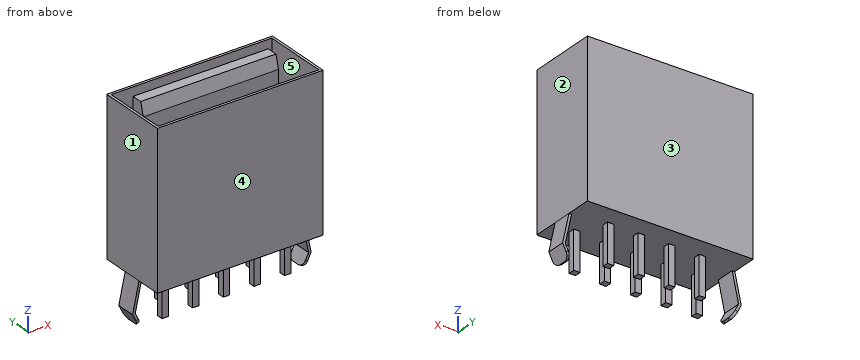
```python
from build123d import *

# Parameters (mm, degrees)
SKETCH_1_W          = 13
SKETCH_1_H          = 5.5
EXTRUDE_1_DEPTH     = 12
SKETCH_2_W          = 12.6
SKETCH_2_H          = 5.1
CUT_EXTRUDE_1_DEPTH = 10
SKETCH_5_W          = 10.6
SKETCH_5_H          = 1.1
EXTRUDE_3_DEPTH     = 10
CHAMFER_1_SIZE      = 1
CHAMFER_1_SIZE2     = 0.267949192
SKETCH_13_W         = 0.5
SKETCH_13_H         = 0.5
EXTRUDE_7_DEPTH     = 3
THICKEN_START       = -0.75
THICKEN_1_DEPTH     = 1.5
THICKEN_2_DEPTH     = 1.5
FILLET_2_R          = 0.5


# Read off the part's stored shape, not the designer's step: 加厚1, 加厚2
with BuildPart() as part:
    # 草图1 → 凸台-拉伸1 (new body)
    with BuildSketch(Plane.XY):
        Rectangle(SKETCH_1_W, SKETCH_1_H)
    extrude(amount=EXTRUDE_1_DEPTH)

    # 草图2 → 切除-拉伸1 (cut)
    with BuildSketch(Plane.XY.offset(12)):
        Rectangle(SKETCH_2_W, SKETCH_2_H)
    extrude(amount=-CUT_EXTRUDE_1_DEPTH, mode=Mode.SUBTRACT)

    # 草图5 → 凸台-拉伸3 (add)
    with BuildSketch(Plane.XY.offset(2)):
        with Locations((0, 1)):
            Rectangle(SKETCH_5_W, SKETCH_5_H)
    extrude(amount=EXTRUDE_3_DEPTH)

    # 倒角1
    chamfer_1_edges = [part.edges().sort_by_distance(p)[0] for p in [
        (0, 0.45, 12),
    ]]
    chamfer_1_side = [part.faces().sort_by_distance(p)[0] for p in [
        (0, 0.45, 7),
    ]]
    chamfer(chamfer_1_edges, length=CHAMFER_1_SIZE, length2=CHAMFER_1_SIZE2, reference=chamfer_1_side[0])

    # 草图13 → 凸台-拉伸7 (add)
    with BuildSketch(Plane(origin=(0, 0, 0), x_dir=(-1, 0, 0), z_dir=(0, 0, -1))):
        with Locations((-3.6, 1)):
            Rectangle(SKETCH_13_W, SKETCH_13_H)
        with Locations((-1.2, 1)):
            Rectangle(SKETCH_13_W, SKETCH_13_H)
        with Locations((1.2, 1)):
            Rectangle(SKETCH_13_W, SKETCH_13_H)
        with Locations((3.6, 1)):
            Rectangle(SKETCH_13_W, SKETCH_13_H)
        with Locations((-2.4, -0.993127881)):
            Rectangle(SKETCH_13_W, SKETCH_13_H)
        with Locations((-4.8, -0.993127881)):
            Rectangle(SKETCH_13_W, SKETCH_13_H)
        with Locations((0, -0.993127881)):
            Rectangle(SKETCH_13_W, SKETCH_13_H)
        with Locations((2.4, -0.993127881)):
            Rectangle(SKETCH_13_W, SKETCH_13_H)
        with Locations((4.8, -0.993127881)):
            Rectangle(SKETCH_13_W, SKETCH_13_H)
    extrude(amount=EXTRUDE_7_DEPTH)

    # 加厚1 outline → 加厚1 (add)
    with BuildSketch(Plane(origin=(0, 0, 0), x_dir=(1, 0, 0), z_dir=(0, 1, 0)).offset(THICKEN_START)):
        Polygon((6.78959064, 2.273605125), (6.295328656, 0), (6.5, 0), (7, 2.3), (6.5, 3.3), (6.321114562, 3.210557281), align=None)
    extrude(amount=THICKEN_1_DEPTH)

    # 加厚2 outline → 加厚2 (add)
    with BuildSketch(Plane(origin=(0, 0, 0), x_dir=(1, 0, 0), z_dir=(0, 1, 0)).offset(THICKEN_START)):
        Polygon((-6.5, 0), (-6.295328656, 0), (-6.78959064, 2.273605125), (-6.321114562, 3.210557281), (-6.5, 3.3), (-7, 2.3), align=None)
    extrude(amount=THICKEN_2_DEPTH)

    # 圆角2
    fillet_2_edges = [part.edges().sort_by_distance(p)[0] for p in [
        (6.410557281, -0.75, -3.25527864),
        (6.410557281, 0.75, -3.25527864),
        (-6.410557281, -0.75, -3.25527864),
        (-6.410557281, 0.75, -3.25527864),
    ]]
    fillet(fillet_2_edges, radius=FILLET_2_R)


solid = part.part
```
Source: CAD feature listing. Evaluate the final solid. Frame: model axes, mm. Face numbers are marked on the shaded views. A direction names the side the tool comes from. Round coordinates to 2 decimals unless told otherwise and drop trailing zeros. Loops run counter-clockwise (first coordinate to the right, second up) from the corner with the lowest first, then second, coordinate; pieces in that order, holes last.
1. Mould query, pull axis Y, two halves, no side actions, for the marked faces 3, 4 and 5. Classes: released by +Y, released by -Y, zero draft, split by the parting line, or undercut.
2. Access query for the marked faces 1 and 2. Directions: +Z, -Z, +X, -X, +Y, -Y. A direction counts if a zero-diameter tool reaches every point of the face in a straight line with its end or side. Return the directions, or none.
3. Section query C-C on y = -2.35. Output: boundary loops of the cut face in (x, z), and give its area (3 significant figures).
4. Section query B-B on x = 0.5. Output: boundary loops of the cut face in (y, z).
5. Section query A-A on z = 8. Output: boundary loops of the cut face in (x, y).
6. Section query D-D on x = -6. Output: boundary loops of the cut face in (y, z).
7. Contact query for flat-ended pins moving along their axis: pin 1 (0.6 mm diameter, centred on x = 1, z = -2, fed in from -Y); pin 2 (0.6 mm diameter, centred on x = 2.5, z = -1, fed in from +Y); pin 3 (0.6 mm diameter, centred on x = -3.5, y = 1, fed in from -Z). Output: stop coordinate, or through.
8. Ray query, L1, parallel to Y at x = 4.5, z = 5.25; L2, parallel to X at y = 1.1, z = 6. Return the intervals inside material, ascending.
Answers below:
1. face 3: released by +Y
1. face 4: released by -Y
1. face 5: undercut
2. face 1: +Z, -X, +Y, -Y
2. face 2: +Z, +X, +Y, -Y
3. outline: (-6.5, 0) - (6.5, 0) - (6.5, 12) - (6.3, 12) - (6.3, 2) - (-6.3, 2) - (-6.3, 12) - (-6.5, 12) - close
3. area: 30.0 mm2
4. outline: (-2.75, 0) - (2.75, 0) - (2.75, 12) - (2.55, 12) - (2.55, 2) - (1.55, 2) - (1.55, 12) - (0.72, 12) - (0.45, 11) - (0.45, 2) - (-2.55, 2) - (-2.55, 12) - (-2.75, 12) - close
5. outline: (-6.5, -2.75) - (6.5, -2.75) - (6.5, 2.75) - (-6.5, 2.75) - close; (-5.3, 0.45) - (5.3, 0.45) - (5.3, 1.55) - (-5.3, 1.55) - close; hole (-6.3, -2.55) - (6.3, -2.55) - (6.3, 2.55) - (-6.3, 2.55) - close
6. outline: (-2.75, 0) - (2.75, 0) - (2.75, 12) - (2.55, 12) - (2.55, 2) - (-2.55, 2) - (-2.55, 12) - (-2.75, 12) - close
7. pin 1: stops at y = 0.75
7. pin 2: stops at y = -0.74
7. pin 3: stops at z = -3
8. L1: y = -2.75 to -2.55, 0.45 to 1.55, 2.55 to 2.75
8. L2: x = -6.5 to -6.3, -5.3 to 5.3, 6.3 to 6.5
